The listing builds one solid part. Answer for the finished solid, in the listing's coordinates (mm). Face numbers are marked on the shaded views. Coordinates: 2 decimals unless noted, no trailing zeros. Use a Markdown table: item, result. Add a question column.
Item 1: Flat-ended cylindrical pins translate along their axes: P1, Ø6, axis at x = 25, y = -4, coming from the +Z side; P2, Ø3, axis at x = -15.5, y = -2, coming from the -Z side; P3, Ø1.2, axis at x = 2, z = 1, coming from the -Y side. Find the tip coordinate at first contact, or state that the pin passes through.
Item 2: The mould has two halves that part along X. Classify the marked faces 1 and 2: released by +X, released by -X, zero draft, split by the parting line, or undercut.
Item 3: Find the intervals of material crossed by line 1 along Z through (x, y) = (23, -10.75); line 2 along Y through (x, z) = (-28.5, 1.75); line 3 along X through (y, z) = (-8.5, 0.2), in increasing order.
from build123d import *

# Parameters (mm, degrees)
F0_W      = 80
F0_H      = 25
F1_DEPTH  = 1.5
F2_R      = 10
F4_DEPTH  = 80
F3_R      = 1.75
F3_R_2    = 1.25
F5_DEPTH  = 80
F6_DEPTH  = 80
F7_W      = 20
F7_H      = 18.6819097605
F7_H_2    = 7
F8_DEPTH  = 25
F10_DEPTH = 0.5
F11_R     = 0.49999


# Not quite as in the source:
# - a fillet or chamfer is up to 0.001 mm smaller than in the source, because OpenCascade refuses the exact size


with BuildPart() as f1:
    # F0 (on Top) → F1 (new body)
    with BuildSketch(Plane.XY):
        Rectangle(F0_W, F0_H)
    extrude(amount=F1_DEPTH)

    # F2
    f2_edges = [f1.edges().sort_by_distance(p)[0] for p in [
        (-40, 12.5, 0.75),
        (40, 12.5, 0.75),
    ]]
    fillet(f2_edges, radius=F2_R)

    # F3 (on face) → F4 (cut)
    with BuildSketch(Plane(origin=(-40, 0, 0), x_dir=(0, -1, 0), z_dir=(-1, 0, 0))):
        with BuildLine():
            Line((12.5, 1.5), (12.4820508076, 1.5))
            ThreePointArc((12.4820508076, 1.5), (11.8956439237, 0.4271243445), (10.75, 0))
            Line((10.75, 0), (12.5, 0))
            Line((12.5, 0), (12.5, 1.5))
        make_face()
        with BuildLine():
            ThreePointArc((12.4820508076, 1.5), (12.495506934, 1.6246782406), (12.5, 1.75))
            ThreePointArc((12.5, 1.75), (10.6246782406, 3.495506934), (9.0179491924, 1.5))
            Line((9.0179491924, 1.5), (9.5252551286, 1.5))
            ThreePointArc((9.5252551286, 1.5), (10.6243637975, 2.9936701913), (12, 1.75))
            ThreePointArc((12, 1.75), (11.9936701913, 1.6243637975), (11.9747448714, 1.5))
            Line((11.9747448714, 1.5), (12.4820508076, 1.5))
        make_face()
    extrude(amount=-F4_DEPTH, mode=Mode.SUBTRACT)

    # F3 (on face) → F5 (join)
    with BuildSketch(Plane(origin=(-40, 0, 0), x_dir=(0, -1, 0), z_dir=(-1, 0, 0))):
        with Locations((10.75, 1.75)):
            Circle(F3_R)
        with Locations((10.75, 1.75)):
            Circle(F3_R_2, mode=Mode.SUBTRACT)
    extrude(amount=-F5_DEPTH)

    # F3 (on face) → F6 (cut)
    with BuildSketch(Plane(origin=(-40, 0, 0), x_dir=(0, -1, 0), z_dir=(-1, 0, 0))):
        with BuildLine():
            Line((11.9747448714, 1.5), (9.5252551286, 1.5))
            ThreePointArc((9.5252551286, 1.5), (10.75, 0.5), (11.9747448714, 1.5))
        make_face()
        with BuildLine():
            ThreePointArc((12, 1.75), (10.6243637975, 2.9936701913), (9.5252551286, 1.5))
            Line((9.5252551286, 1.5), (11.9747448714, 1.5))
            ThreePointArc((11.9747448714, 1.5), (11.9936701913, 1.6243637975), (12, 1.75))
        make_face()
    extrude(amount=-F6_DEPTH, mode=Mode.SUBTRACT)

    # F7 (on face) → F8 (cut)
    with BuildSketch(Plane(origin=(0, 0, 0), x_dir=(1, 0, 0), z_dir=(0, 0, -1))):
        with Locations((0, 20.0909548802)):
            Rectangle(F7_W, F7_H)
        with Locations((0, 7.25)):
            Rectangle(F7_W, F7_H_2)
    extrude(amount=-F8_DEPTH, mode=Mode.SUBTRACT)

    # F9 (on face) → F10 (join)
    with BuildSketch(Plane(origin=(0, 0, 0), x_dir=(1, 0, 0), z_dir=(0, 0, -1))):
        with BuildLine():
            Line((-36, 8.5), (-37, 8.5))
            Line((-37, 8.5), (-37, 0.5))
            ThreePointArc((-37, 0.5), (-34.0710678119, -6.5710678119), (-27, -9.5))
            Line((-27, -9.5), (-7, -9.5))
            Line((-7, -9.5), (-7, 0.5))
            Line((-7, 0.5), (-8, 0.5))
            Line((-8, 0.5), (-8, -8.5))
            Line((-8, -8.5), (-27, -8.5))
            ThreePointArc((-27, -8.5), (-33.3639610307, -5.8639610307), (-36, 0.5))
            Line((-36, 0.5), (-36, 8.5))
        make_face()
        with BuildLine():
            Line((8, 0.5), (7, 0.5))
            Line((7, 0.5), (7, -9.5))
            Line((7, -9.5), (27, -9.5))
            ThreePointArc((27, -9.5), (34.0710678119, -6.5710678119), (37, 0.5))
            Line((37, 0.5), (37, 8.5))
            Line((37, 8.5), (36, 8.5))
            Line((36, 8.5), (36, 0.5))
            ThreePointArc((36, 0.5), (33.3639610307, -5.8639610307), (27, -8.5))
            Line((27, -8.5), (8, -8.5))
            Line((8, -8.5), (8, 0.5))
        make_face()
    extrude(amount=F10_DEPTH)

    # F11 (radius 0.5 in the source; OpenCascade refuses exactly that, so slightly less here)
    f11_edges = [f1.edges().sort_by_distance(p)[0] for p in [
        (-36, -4.5, -0.5),
        (-36.5, -8.5, -0.5),
        (-37, -4.5, -0.5),
        (-34.071068, 6.571068, -0.5),
        (-17, 9.5, -0.5),
        (-7, 4.5, -0.5),
        (-7.5, -0.5, -0.5),
        (-8, 4, -0.5),
        (-17.5, 8.5, -0.5),
        (-33.363961, 5.863961, -0.5),
        (17.5, 8.5, -0.5),
        (8, 4, -0.5),
        (7.5, -0.5, -0.5),
        (7, 4.5, -0.5),
        (17, 9.5, -0.5),
        (34.071068, 6.571068, -0.5),
        (37, -4.5, -0.5),
        (36.5, -8.5, -0.5),
        (36, -4.5, -0.5),
        (33.363961, 5.863961, -0.5),
    ]]
    fillet(f11_edges, radius=F11_R)


solid = f1.part
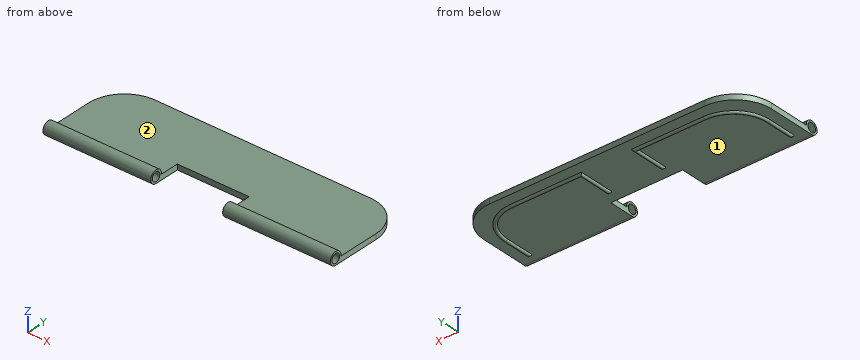
Solution:
| question | item | result |
|---|---|---|
| 1 | P1 | stops at z = 1.5 |
| 1 | P2 | stops at z = 0 |
| 1 | P3 | stops at y = -3.75 |
| 2 | face 1 | undercut |
| 2 | face 2 | zero draft |
| 3 | line 1 | z = 0 to 0.5, 3 to 3.5 |
| 3 | line 2 | y = -12.5 to -12, -9.5 to -9 |
| 3 | line 3 | x = -40 to -10, 10 to 40 |
